The model under review builds one solid part; all positions refer to its coordinate system, in mm. A direction names the side the tool comes from. Coordinates: 2 decimals unless noted, no trailing zeros. Loops run counter-clockwise (first coordinate to the right, second up) from the corner with the lowest first, then second, coordinate; pieces in that order, holes last. Notation, with made-up numbers: (40, 7.5) - (81, 7.5) arc R25 ccw to (81, 45.5) - close; hole circle Ø4 at (-40, 54). An arc over 180 degrees is marked (long way). One line per item, written item: value. Start each with the question number.
1. We need section B-B, the plane x = 28.5. Give the boundary of the cut face in (y, z), then the cut area to 3 significant figures.
2. We need section D-D, the plane x = 19. Give the boundary of the cut face in (y, z).
3. Insertion check: P1, Ø3.5, axis at y = 12.5, z = 12, coming from the +X side. The pin has a flat end and moves straight along its axis. Give the tip position at first contact, or say it passes through.
4. For faces 1 (the face through (0, 0, 0)), 2 (the face through (27, 12, 12)), 3 (the face through (18.619, 11.648, 20.944)), 4 (the face through (22, 13, 7)), 5 (the face through (8, 15, 5)), list the 3-axis set-ups (+Z, -Z, +X, -X, +Y, -Y) from which the entire face can be reached by the end or side of a thin tool; tool diameter is ignored.
5. We need section C-C, the plane y = 3.75. Give the boundary of the cut face in (x, z) (3 decimals), then the cut area to 3 significant figures.
6. We need section A-A, the plane z = 19. Give the boundary of the cut face in (x, y), then the cut area to 3 significant figures.
7. To check wall thickness, follow line 1 (Y direction, x = 20.5, z = 22.5); line 2 (Y direction, x = 29, z = -19.5); line 3 (X direction, y = 13.25, z = 0) (3 decimals). State the ranges of each line that lie inside material, in increasing order.
from build123d import *

# Parameters (mm, degrees)
SKETCH_1_W          = 50
SKETCH_1_H          = 30
EXTRUDE_1_DEPTH     = 40
CUT_EXTRUDE_1_DEPTH = 66.76473219
CUT_EXTRUDE_2_DEPTH = 56.901699437
SKETCH_4_W          = 17
SKETCH_4_H          = 6.8
CUT_EXTRUDE_3_DEPTH = 18
EXTRUDE_2_REACH     = 57.902
EXTRUDE_4_REACH     = 57.902


with BuildPart() as part:
    # Эскиз1 → Бобышка-Вытянуть1 (new body)
    with BuildSketch(Plane(origin=(0, 0, 0), x_dir=(0, 0, -1), z_dir=(1, 0, 0))):
        Rectangle(SKETCH_1_W, SKETCH_1_H)
    extrude(amount=EXTRUDE_1_DEPTH)

    # Эскиз2 → Вырез-Вытянуть1 (cut, through all)
    with BuildSketch(Plane.XY.offset(25)):
        Polygon((10, 15), (40, 3), (40, 15), align=None)
    extrude(amount=-CUT_EXTRUDE_1_DEPTH, mode=Mode.SUBTRACT)

    # Эскиз3 → Вырез-Вытянуть2 (cut, through all)
    with BuildSketch(Plane.XZ.offset(15)):
        Polygon((40, 13), (27, 25), (40, 25), align=None)
    extrude(amount=-CUT_EXTRUDE_2_DEPTH, mode=Mode.SUBTRACT)

    # Эскиз4 → Вырез-Вытянуть3 (cut)
    with BuildSketch(Plane.XY.offset(25)):
        with Locations((18.5, 11.6)):
            Rectangle(SKETCH_4_W, SKETCH_4_H)
    extrude(amount=-CUT_EXTRUDE_3_DEPTH, mode=Mode.SUBTRACT)

    # Бобышка-Вытянуть2: up to this face of the body (flat: up to its plane)
    extrude_2_end = Plane(part.part.faces().sort_by_distance((18.5, 8.2, 16))[0])
    # Эскиз5 → Бобышка-Вытянуть2 (add, up to the picked face)
    with BuildSketch(Plane(origin=(0, 15, 0), x_dir=(1, 0, 0), z_dir=(0, 1, 0)), mode=Mode.PRIVATE) as extrude_2_sk1:
        Polygon((10, -7), (27, -7), (27, -17), (10, -25), align=None)
    extrude_2_tool1 = split(extrude(extrude_2_sk1.sketch, amount=-EXTRUDE_2_REACH, mode=Mode.PRIVATE), bisect_by=extrude_2_end, keep=Keep.BOTH, mode=Mode.PRIVATE)
    add(extrude_2_tool1.solids().sort_by(Axis((17.690476, 15, 14.190476), (0, -1, 0)))[0])

    # Бобышка-Вытянуть4: up to this face of the body (flat: up to its plane)
    extrude_4_end = Plane(part.part.faces().sort_by_distance((26.036738351, 8.585304659, -5.85483871))[0])
    # Эскиз6 → Бобышка-Вытянуть4 (add, up to the picked face)
    with BuildSketch(Plane.XZ.offset(15), mode=Mode.PRIVATE) as extrude_4_sk1:
        Polygon((27, 25), (40, 13), (40, 25), align=None)
    extrude_4_tool1 = split(extrude(extrude_4_sk1.sketch, amount=-EXTRUDE_4_REACH, mode=Mode.PRIVATE), bisect_by=extrude_4_end, keep=Keep.BOTH, mode=Mode.PRIVATE)
    add(extrude_4_tool1.solids().sort_by(Axis((35.666667, -15, 21), (0, 1, 0)))[0])


solid = part.part
Findings below:
1. outline: (-15, -25) - (7.6, -25) - (7.6, 25) - (-15, 25) - close
1. area: 1,130 mm2
2. outline: (-15, -25) - (11.4, -25) - (11.4, 7) - (15, 7) - (15, 20.76) - (8.2, 20.76) - (8.2, 25) - (-15, 25) - close
3. P1: x = 27
4. face 1: +Z, -Z, -X, +Y, -Y
4. face 2: +Z, -Z, +X, +Y
4. face 3: +Z, +X, +Y
4. face 4: -Z, +X, +Y
4. face 5: +Z, -Z, +X, -X, +Y
5. outline: (0, -25) - (38.125, -25) - (38.125, 25) - (0, 25) - close
5. area: 1,910 mm2
6. outline: (0, -15) - (40, -15) - (40, 3) - (27, 8.2) - (22.75, 8.2) - (22.75, 15) - (0, 15) - close
6. area: 1,050 mm2
7. line 1: -15 to 8.2
7. line 2: -15 to 7.4
7. line 3: 0 to 14.375
